```python
from build123d import *

# Parameters (mm, degrees)
SKETCH_1_W           = 70
SKETCH_1_H           = 30
EXTRUDE_1_DEPTH      = 9
SKETCH_2_W           = 112.1
SKETCH_2_H           = 30
EXTRUDE_2_DEPTH      = 8
SKETCH_3_W           = 42.6
SKETCH_3_H           = 30
EXTRUDE_3_DEPTH      = 8
SKETCH_5_W           = 18.5
SKETCH_5_H           = 30
SKETCH_5_R           = 2
EXTRUDE_4_DEPTH      = 5.5
SKETCH_11_R          = 2
CUT_EXTRUDE_4_DEPTH  = 8
SKETCH_12_R          = 1.8
CUT_EXTRUDE_6_DEPTH  = 8
SKETCH_13_R          = 2
CUT_EXTRUDE_7_DEPTH  = 8
SKETCH_14_R          = 2
CUT_EXTRUDE_8_DEPTH  = 10
SKETCH_19_W          = 5
SKETCH_19_H          = 9
EXTRUDE_6_DEPTH      = 36.25
SKETCH_20_W          = 5
SKETCH_20_H          = 6.25
EXTRUDE_7_DEPTH      = 9
SKETCH_21_R          = 1.3
CUT_EXTRUDE_10_DEPTH = 9
SKETCH_25_W          = 5
SKETCH_25_H          = 1.5
EXTRUDE_8_DEPTH      = 42.5
SKETCH_26_R          = 1.3
CUT_EXTRUDE_14_DEPTH = 1.5
SKETCH_27_W          = 5
SKETCH_27_H          = 6.25
CUT_EXTRUDE_15_DEPTH = 11
SKETCH_28_R          = 3
CUT_EXTRUDE_16_DEPTH = 3
SKETCH_29_W          = 8
SKETCH_29_H          = 103.1
SKETCH_29_W_2        = 10.5
SKETCH_29_H_2        = 5.5
CUT_EXTRUDE_17_DEPTH = 30
SKETCH_30_R          = 1.8
CUT_EXTRUDE_18_DEPTH = 10
SKETCH_31_R          = 3.6
CUT_EXTRUDE_19_DEPTH = 3
SKETCH_32_R          = 1.8
CUT_EXTRUDE_20_DEPTH = 10
SKETCH_33_R          = 3.6
CUT_EXTRUDE_21_DEPTH = 3
CUT_EXTRUDE_22_REACH = 86.054
SKETCH_35_R          = 1.8


with BuildPart() as part:
    # 草圖1 → 填料-伸長1 (new body)
    with BuildSketch(Plane.XY):
        with Locations((35, 15)):
            Rectangle(SKETCH_1_W, SKETCH_1_H)
    extrude(amount=EXTRUDE_1_DEPTH)

    # 草圖2 → 填料-伸長2 (add)
    with BuildSketch(Plane.ZY):
        with Locations((-47.05, 15)):
            Rectangle(SKETCH_2_W, SKETCH_2_H)
    extrude(amount=EXTRUDE_2_DEPTH)

    # 草圖3 → 填料-伸長3 (add)
    with BuildSketch(Plane(origin=(70, 0, 0), x_dir=(0, 0, -1), z_dir=(1, 0, 0))):
        with Locations((12.3, 15)):
            Rectangle(SKETCH_3_W, SKETCH_3_H)
    extrude(amount=EXTRUDE_3_DEPTH)

    # 草圖5 → 填料-伸長4 (add)
    with BuildSketch(Plane(origin=(0, 0, -33.6), x_dir=(-1, 0, 0), z_dir=(0, 0, -1))):
        with Locations((-68.75, 15)):
            Rectangle(SKETCH_5_W, SKETCH_5_H)
        with Locations(Location((-65.75, 26, 0), (0, 0, 90))):
            Circle(SKETCH_5_R, mode=Mode.SUBTRACT)
        with Locations(Location((-65.75, 18, 0), (0, 0, 90))):
            Circle(SKETCH_5_R, mode=Mode.SUBTRACT)
        with Locations(Location((-65.75, 10, 0), (0, 0, 90))):
            Circle(SKETCH_5_R, mode=Mode.SUBTRACT)
    extrude(amount=EXTRUDE_4_DEPTH)

    # 草圖11 → 除料-伸長4 (cut)
    with BuildSketch(Plane.ZY.offset(8)):
        with Locations((-23, 23)):
            Circle(SKETCH_11_R)
        with Locations((-23, 15)):
            Circle(SKETCH_11_R)
        with Locations((-23, 7)):
            Circle(SKETCH_11_R)
        with Locations((-15, 23)):
            Circle(SKETCH_11_R)
        with Locations((-15, 15)):
            Circle(SKETCH_11_R)
        with Locations((-15, 7)):
            Circle(SKETCH_11_R)
        with Locations((-7, 23)):
            Circle(SKETCH_11_R)
        with Locations((-7, 15)):
            Circle(SKETCH_11_R)
        with Locations((-7, 7)):
            Circle(SKETCH_11_R)
    extrude(amount=-CUT_EXTRUDE_4_DEPTH, mode=Mode.SUBTRACT)

    # 草圖12 → 除料-伸長6 (cut)
    with BuildSketch(Plane(origin=(0, 0, -103.1), x_dir=(-1, 0, 0), z_dir=(0, 0, -1))):
        with Locations((3, 23)):
            Circle(SKETCH_12_R)
        with Locations((3, 15)):
            Circle(SKETCH_12_R)
        with Locations((3, 7)):
            Circle(SKETCH_12_R)
    extrude(amount=-CUT_EXTRUDE_6_DEPTH, mode=Mode.SUBTRACT)

    # 草圖13 → 除料-伸長7 (cut)
    with BuildSketch(Plane(origin=(78, 0, 0), x_dir=(0, 0, -1), z_dir=(1, 0, 0))):
        with Locations((9.1, 23)):
            Circle(SKETCH_13_R)
        with Locations((9.1, 15)):
            Circle(SKETCH_13_R)
        with Locations((9.1, 7)):
            Circle(SKETCH_13_R)
        with Locations((17.1, 23)):
            Circle(SKETCH_13_R)
        with Locations((17.1, 15)):
            Circle(SKETCH_13_R)
        with Locations((17.1, 7)):
            Circle(SKETCH_13_R)
        with Locations((25.1, 23)):
            Circle(SKETCH_13_R)
        with Locations((25.1, 15)):
            Circle(SKETCH_13_R)
        with Locations((25.1, 7)):
            Circle(SKETCH_13_R)
    extrude(amount=-CUT_EXTRUDE_7_DEPTH, mode=Mode.SUBTRACT)

    # 草圖14 → 除料-伸長8 (cut)
    with BuildSketch(Plane.ZY.offset(8)):
        with Locations((-85.1, 23)):
            Circle(SKETCH_14_R)
        with Locations((-85.1, 15)):
            Circle(SKETCH_14_R)
        with Locations((-85.1, 7)):
            Circle(SKETCH_14_R)
        with Locations((-77.1, 23)):
            Circle(SKETCH_14_R)
        with Locations((-77.1, 15)):
            Circle(SKETCH_14_R)
        with Locations((-77.1, 7)):
            Circle(SKETCH_14_R)
        with Locations((-69.1, 23)):
            Circle(SKETCH_14_R)
        with Locations((-69.1, 15)):
            Circle(SKETCH_14_R)
        with Locations((-69.1, 7)):
            Circle(SKETCH_14_R)
        with Locations((-61.1, 23)):
            Circle(SKETCH_14_R)
        with Locations((-61.1, 15)):
            Circle(SKETCH_14_R)
        with Locations((-61.1, 7)):
            Circle(SKETCH_14_R)
    extrude(amount=-CUT_EXTRUDE_8_DEPTH, mode=Mode.SUBTRACT)

    # 草圖19 → 填料-伸長6 (add)
    with BuildSketch(Plane(origin=(0, 30, 0), x_dir=(1, 0, 0), z_dir=(0, 1, 0))):
        with Locations((22.1, -4.5)):
            Rectangle(SKETCH_19_W, SKETCH_19_H)
        with Locations((48.1, -4.5)):
            Rectangle(SKETCH_19_W, SKETCH_19_H)
    extrude(amount=-EXTRUDE_6_DEPTH)

    # 草圖20 → 填料-伸長7 (add)
    with BuildSketch(Plane(origin=(0, 0, 0), x_dir=(-1, 0, 0), z_dir=(0, 0, -1))):
        with Locations((-48.1, 33.125)):
            Rectangle(SKETCH_20_W, SKETCH_20_H)
        with Locations((-22.1, 33.125)):
            Rectangle(SKETCH_20_W, SKETCH_20_H)
    extrude(amount=-EXTRUDE_7_DEPTH)

    # 草圖21 → 除料-伸長10 (cut)
    with BuildSketch(Plane(origin=(0, 0, 0), x_dir=(-1, 0, 0), z_dir=(0, 0, -1))):
        with Locations((-48.1, 23.75)):
            Circle(SKETCH_21_R)
        with Locations((-48.1, 13.75)):
            Circle(SKETCH_21_R)
        with Locations((-48.1, 3.75)):
            Circle(SKETCH_21_R)
        with Locations((-22.1, 23.75)):
            Circle(SKETCH_21_R)
        with Locations((-22.1, 13.75)):
            Circle(SKETCH_21_R)
        with Locations((-22.1, 3.75)):
            Circle(SKETCH_21_R)
    extrude(amount=-CUT_EXTRUDE_10_DEPTH, mode=Mode.SUBTRACT)

    # 草圖25 → 填料-伸長8 (add)
    with BuildSketch(Plane(origin=(0, 36.25, 0), x_dir=(1, 0, 0), z_dir=(0, 1, 0))):
        with Locations((22.1, 0.75)):
            Rectangle(SKETCH_25_W, SKETCH_25_H)
        with Locations((48.1, 0.75)):
            Rectangle(SKETCH_25_W, SKETCH_25_H)
    extrude(amount=-EXTRUDE_8_DEPTH)

    # 草圖26 → 除料-伸長14 (cut)
    with BuildSketch(Plane(origin=(0, 0, -1.5), x_dir=(-1, 0, 0), z_dir=(0, 0, -1))):
        with Locations((-48.1, 23.75)):
            Circle(SKETCH_26_R)
        with Locations((-48.1, 13.75)):
            Circle(SKETCH_26_R)
        with Locations((-48.1, 3.75)):
            Circle(SKETCH_26_R)
        with Locations((-22.1, 23.75)):
            Circle(SKETCH_26_R)
        with Locations((-22.1, 13.75)):
            Circle(SKETCH_26_R)
        with Locations((-22.1, 3.75)):
            Circle(SKETCH_26_R)
    extrude(amount=-CUT_EXTRUDE_14_DEPTH, mode=Mode.SUBTRACT)

    # 草圖27 → 除料-伸長15 (cut)
    with BuildSketch(Plane.XY.offset(9)):
        with Locations((22.1, 33.125)):
            Rectangle(SKETCH_27_W, SKETCH_27_H)
        with Locations((48.1, 33.125)):
            Rectangle(SKETCH_27_W, SKETCH_27_H)
        with Locations((22.1, -3.125)):
            Rectangle(SKETCH_27_W, SKETCH_27_H)
        with Locations((48.1, -3.125)):
            Rectangle(SKETCH_27_W, SKETCH_27_H)
    extrude(amount=-CUT_EXTRUDE_15_DEPTH, mode=Mode.SUBTRACT)

    # 草圖28 → 除料-伸長16 (cut)
    with BuildSketch(Plane.XY.offset(9)):
        with Locations((22.1, 23.75)):
            Circle(SKETCH_28_R)
        with Locations((22.1, 13.75)):
            Circle(SKETCH_28_R)
        with Locations((22.1, 3.75)):
            Circle(SKETCH_28_R)
        with Locations((48.1, 13.75)):
            Circle(SKETCH_28_R)
        with Locations((48.1, 3.75)):
            Circle(SKETCH_28_R)
        with Locations((48.1, 23.75)):
            Circle(SKETCH_28_R)
    extrude(amount=-CUT_EXTRUDE_16_DEPTH, mode=Mode.SUBTRACT)

    # 草圖29 → 除料-伸長17 (cut)
    with BuildSketch(Plane(origin=(0, 30, 0), x_dir=(1, 0, 0), z_dir=(0, 1, 0))):
        with Locations((-4, 51.55)):
            Rectangle(SKETCH_29_W, SKETCH_29_H)
        with Locations((64.75, 36.35)):
            Rectangle(SKETCH_29_W_2, SKETCH_29_H_2)
        Polygon((70, 33.6), (70, 0), (78, 0), (78, 39.1), (70, 39.1), align=None)
    extrude(amount=-CUT_EXTRUDE_17_DEPTH, mode=Mode.SUBTRACT)

    # 草圖30 → 除料-伸長18 (cut)
    with BuildSketch(Plane.XY.offset(9)):
        with Locations((-4, 23)):
            Circle(SKETCH_30_R)
        with Locations((-4, 15)):
            Circle(SKETCH_30_R)
        with Locations((-4, 7)):
            Circle(SKETCH_30_R)
    extrude(amount=-CUT_EXTRUDE_18_DEPTH, mode=Mode.SUBTRACT)

    # 草圖31 → 除料-伸長19 (cut)
    with BuildSketch(Plane.XY.offset(9)):
        with Locations((-4, 15)):
            Circle(SKETCH_31_R)
        with Locations((-4, 7)):
            Circle(SKETCH_31_R)
        with Locations((-4, 23)):
            Circle(SKETCH_31_R)
    extrude(amount=-CUT_EXTRUDE_19_DEPTH, mode=Mode.SUBTRACT)

    # 草圖32 → 除料-伸長20 (cut)
    with BuildSketch(Plane.XY.offset(9)):
        with Locations((74, 23)):
            Circle(SKETCH_32_R)
        with Locations((74, 15)):
            Circle(SKETCH_32_R)
        with Locations((74, 7)):
            Circle(SKETCH_32_R)
    extrude(amount=-CUT_EXTRUDE_20_DEPTH, mode=Mode.SUBTRACT)

    # 草圖33 → 除料-伸長21 (cut)
    with BuildSketch(Plane.XY.offset(9)):
        with Locations((74, 23)):
            Circle(SKETCH_33_R)
        with Locations((74, 15)):
            Circle(SKETCH_33_R)
        with Locations((74, 7)):
            Circle(SKETCH_33_R)
    extrude(amount=-CUT_EXTRUDE_21_DEPTH, mode=Mode.SUBTRACT)

    # 草圖35 → 除料-伸長22 (cut, up to next)
    with BuildSketch(Plane(origin=(0, 0, 0), x_dir=(-1, 0, 0), z_dir=(0, 0, -1)), mode=Mode.PRIVATE) as cut_extrude_22_sk1:
        with Locations((-43.1, 4)):
            Circle(SKETCH_35_R)
    cut_extrude_22_tool1 = extrude(cut_extrude_22_sk1.sketch, amount=-CUT_EXTRUDE_22_REACH, mode=Mode.PRIVATE) & part.part
    # 草圖35 → 除料-伸長22 (cut, up to next)
    with BuildSketch(Plane(origin=(0, 0, 0), x_dir=(-1, 0, 0), z_dir=(0, 0, -1)), mode=Mode.PRIVATE) as cut_extrude_22_sk2:
        with Locations((-43.1, 26)):
            Circle(SKETCH_35_R)
    cut_extrude_22_tool2 = extrude(cut_extrude_22_sk2.sketch, amount=-CUT_EXTRUDE_22_REACH, mode=Mode.PRIVATE) & part.part
    # 草圖35 → 除料-伸長22 (cut, up to next)
    with BuildSketch(Plane(origin=(0, 0, 0), x_dir=(-1, 0, 0), z_dir=(0, 0, -1)), mode=Mode.PRIVATE) as cut_extrude_22_sk3:
        with Locations((-27.1, 26)):
            Circle(SKETCH_35_R)
    cut_extrude_22_tool3 = extrude(cut_extrude_22_sk3.sketch, amount=-CUT_EXTRUDE_22_REACH, mode=Mode.PRIVATE) & part.part
    # 草圖35 → 除料-伸長22 (cut, up to next)
    with BuildSketch(Plane(origin=(0, 0, 0), x_dir=(-1, 0, 0), z_dir=(0, 0, -1)), mode=Mode.PRIVATE) as cut_extrude_22_sk4:
        with Locations((-27.1, 4)):
            Circle(SKETCH_35_R)
    cut_extrude_22_tool4 = extrude(cut_extrude_22_sk4.sketch, amount=-CUT_EXTRUDE_22_REACH, mode=Mode.PRIVATE) & part.part
    add(cut_extrude_22_tool1.solids().sort_by_distance((43.1, 4, 0))[0], mode=Mode.SUBTRACT)
    add(cut_extrude_22_tool2.solids().sort_by_distance((43.1, 26, 0))[0], mode=Mode.SUBTRACT)
    add(cut_extrude_22_tool3.solids().sort_by_distance((27.1, 26, 0))[0], mode=Mode.SUBTRACT)
    add(cut_extrude_22_tool4.solids().sort_by_distance((27.1, 4, 0))[0], mode=Mode.SUBTRACT)


solid = part.part
```
The model under review builds one solid part; all positions refer to its coordinate system, in mm. A direction names the side the tool comes from. Round coordinates to 2 decimals unless told otherwise and drop trailing zeros. Write each loop counter-clockwise with the first axis right and the second up, starting at its lowest first coordinate (ties: lowest second). Pieces come first, ordered by that corner, then holes.
(1) Mouldability with a two-part tool opening along Y and no side actions: class faces 4 (the flat face through (-8, 15, 4)), 5 (the cylindrical face through (72.572, 5.905, 3.042)) as +Y half, -Y half, draft (parallel to the pull), parting line (faces both ways), or undercut.
(2) We need section B-B on x = 43.1. Give the boundary of the cut face in (y, z).
(3) Machinability: for faces 1 (the cylindrical face through (47.5, 22.597, 2.198)), 2 (the flat face through (45.6, 15, -1)), 3 (the cylindrical face through (75.661, 11.806, 7.521)), which of the approach directions +Z, -Z, +X, -X, +Y, -Y give a long, thin tool a straight path to every point of the face, cutting with its end or side? Answer none if there is none.
(4) We need section C-C on x = -4. Give the boundary of the cut face in (y, z), and give its area (3 significant figures).
(5) We need section A-A on z = 6.75. Give the number of separate pieces and of enclosed holes in the cut face, and give its area (3 significant figures).
(6) Insertion check: pin 1 (0.8 mm diameter, centred on y = 11.5, z = -0.5, fed in from -X); pin 2 (1.5 mm diameter, centred on x = 18, y = 22, fed in from -Z); pin 3 (5.5 mm diameter, centred on x = 22.1, y = 13.75, fed in from +Z); pin 4 (9.5 mm diameter, centred on x = 22.1, y = 3.75, fed in from +Z). Each pin has a flat end and moves straight along its axis. Give the tip position at first contact, or say it passes through.
(7) Wall thickness on L1, parallel to Y at x = 22.1, z = 3.25; L2, parallel to Y at x = 27.1, z = 4.5; L3, parallel to Y at x = -4, z = 3.2: over which ranges is each line inside the solid? List them lowest first.
Findings below:
1. face 4: draft
1. face 5: undercut
2. outline: (0, 0) - (2.2, 0) - (2.2, 9) - (0, 9) - close; (5.8, 0) - (24.2, 0) - (24.2, 9) - (5.8, 9) - close; (27.8, 0) - (30, 0) - (30, 9) - (27.8, 9) - close
3. face 1: +Z, -Z
3. face 2: -Z, +Y, -Y
3. face 3: +Z
4. outline: (0, 0) - (5.2, 0) - (5.2, 6) - (3.4, 6) - (3.4, 9) - (0, 9) - close; (8.8, 0) - (13.2, 0) - (13.2, 6) - (11.4, 6) - (11.4, 9) - (10.6, 9) - (10.6, 6) - (8.8, 6) - close; (16.8, 0) - (21.2, 0) - (21.2, 6) - (19.4, 6) - (19.4, 9) - (18.6, 9) - (18.6, 6) - (16.8, 6) - close; (24.8, 0) - (30, 0) - (30, 9) - (26.6, 9) - (26.6, 6) - (24.8, 6) - close
4. area: 140 mm2
5. separate pieces: 1
5. enclosed holes: 16
5. area: 2,130 mm2
6. pin 1: stops at x = 19.6
6. pin 2: stops at z = 0
6. pin 3: stops at z = 6
6. pin 4: stops at z = 9
7. L1: y = 0 to 2.45, 5.05 to 12.45, 15.05 to 22.45, 25.05 to 30
7. L2: y = 0 to 2.2, 5.8 to 24.2, 27.8 to 30
7. L3: y = 0 to 5.2, 8.8 to 13.2, 16.8 to 21.2, 24.8 to 30
